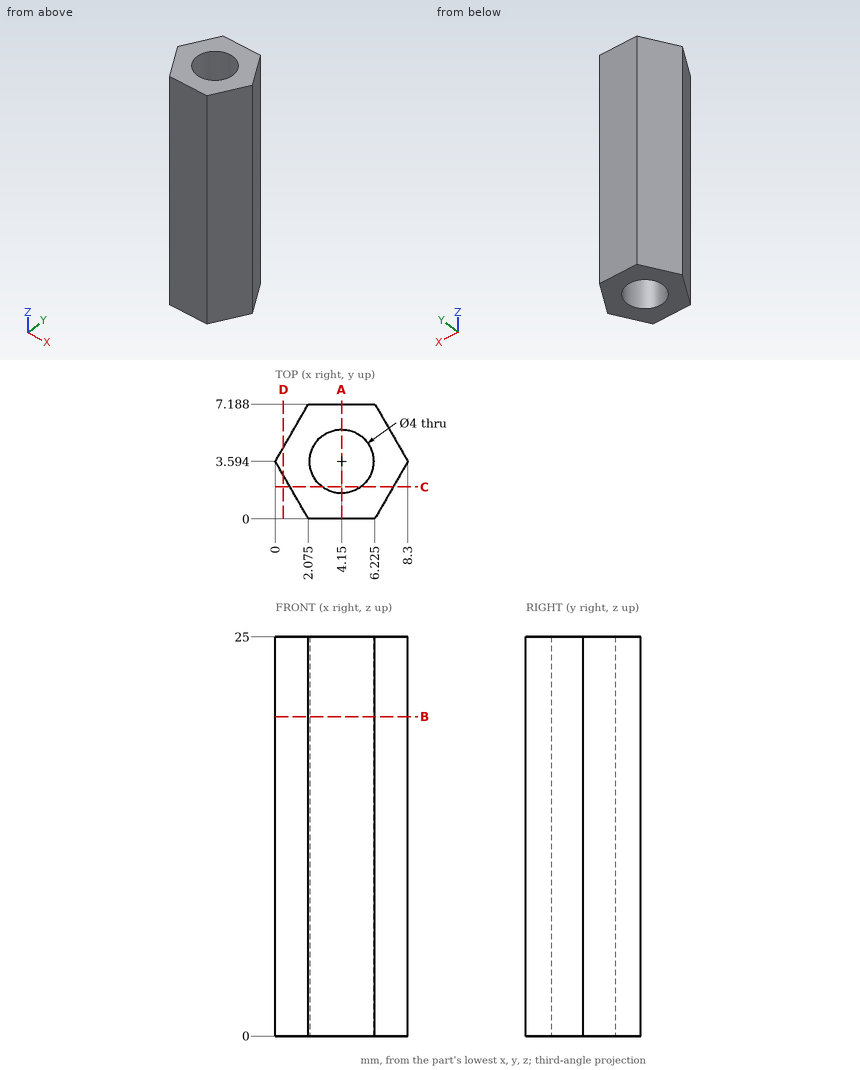
Here's the drawing with two shaded views (mm, measured from the low corner). I have some questions. Give positions to 0.01 mm unless a question says otherwise; leave off trailing zeros. Loops run counter-clockwise (first coordinate to the right, second up) from the corner with the lowest first, then second, coordinate; pieces in that order, holes last. Notation, with made-up numbers: (-17.75, 1) -> (0.25, 1) arc R34 cw to (0.25, 33) -> close; hole circle Ø2 at (74.25, 38.25). An arc over 180 degrees is marked (long way). One line per item, written item: value.
Q1. Suppose I cut it at B-B on z = 20. Please give me the cut outline in (x, y) (3 decimals), then the cut area to 3 significant figures.
Answers follow:
outline: (0, 3.594) -> (2.075, 0) -> (6.225, 0) -> (8.3, 3.594) -> (6.225, 7.188) -> (2.075, 7.188) -> close; hole circle Ø4 at (4.15, 3.594)
area: 32.2 mm^2
Q2. Suppose I cut it at A-A on x = 4.15. Please give me the cut outline in (y, z).
Answers follow:
outline: (0, 0) -> (1.59, 0) -> (1.59, 25) -> (0, 25) -> close; (5.59, 0) -> (7.19, 0) -> (7.19, 25) -> (5.59, 25) -> close
Q3. Suppose I cut it at C-C on y = 2. Please give me the cut outline in (x, z), then the cut area to 3 significant figures.
Answers follow:
outline: (0.92, 0) -> (2.94, 0) -> (2.94, 25) -> (0.92, 25) -> close; (5.36, 0) -> (7.38, 0) -> (7.38, 25) -> (5.36, 25) -> close
area: 101 mm^2
Q4. Suppose I cut it at D-D on x = 0.5. Please give me the cut outline in (y, z).
Answers follow:
outline: (2.73, 0) -> (4.46, 0) -> (4.46, 25) -> (2.73, 25) -> close
Q5. If I drill on line 1 along Y through (x, z) = (4.15, 16.5); line 2 along X through (y, z) = (4, 7); line 3 along Y through (x, z) = (5.75, 7.25), over which ranges is the centre line in solid material (lowest first)?
Answers follow:
line 1: 0 to 1.59, 5.59 to 7.19
line 2: 0.23 to 2.19, 6.11 to 8.07
line 3: 0 to 2.39, 4.79 to 7.19
Q6. I'm going to push flat-ended pins straight in: pin 1 Ø1 at (x, y) = (5, 4) entering from +Z; pin 2 Ø4 at (y, z) = (6, 22.5) entering from +X; pin 3 Ø2 at (y, z) = (1.5, 20.5) entering from -X. Where does each tip first touch, or does it pass through?
Answers follow:
pin 1: through
pin 2: x = 8.07
pin 3: x = 0.63
